Geometry check sheet. Reference: the model listing, model coordinates, mm. A direction names the side the tool comes from. Give positions to 0.01 mm unless a question says otherwise; leave off trailing zeros. Loops run counter-clockwise (first coordinate to the right, second up) from the corner with the lowest first, then second, coordinate; pieces in that order, holes last. Notation, with made-up numbers: (-37, 34.5) -> (-8, 34.5) arc R26 ccw to (-8, 61.5) -> close; hole circle Ø9 at (40, 34). An arc over 180 degrees is marked (long way). Write item = value, one per line.
```python
from build123d import *

# Parameters (mm, degrees)
SKETCH1_W           = 19.05
SKETCH1_H           = 25.4
BOSS_EXTRUDE1_DEPTH = 6.35
SKETCH2_W           = 6.35
SKETCH2_H           = 6.35
CUT_EXTRUDE1_DEPTH  = 7.35
SKETCH6_R           = 0.635
CUT_EXTRUDE2_DEPTH  = 7.35
SKETCH7_R           = 0.635
CUT_EXTRUDE3_DEPTH  = 7.35


with BuildPart() as part:
    # Sketch1 → Boss-Extrude1 (new body)
    with BuildSketch(Plane.XY):
        with Locations((9.525, 12.7)):
            Rectangle(SKETCH1_W, SKETCH1_H)
    extrude(amount=BOSS_EXTRUDE1_DEPTH)

    # Sketch2 → Cut-Extrude1 (cut, through all)
    with BuildSketch(Plane.XY.offset(6.35)):
        with Locations((9.525, 22.225)):
            Rectangle(SKETCH2_W, SKETCH2_H)
    cut_extrude1 = extrude(amount=-CUT_EXTRUDE1_DEPTH, mode=Mode.SUBTRACT)

    # Mirror1: Cut-Extrude1 across plane
    add(cut_extrude1.mirror(Plane.ZX.offset(12.7)), mode=Mode.SUBTRACT)

    # Sketch6 → Cut-Extrude2 (cut, through all)
    with BuildSketch(Plane.XY.offset(6.35)):
        with Locations((3.175, 22.225)):
            Circle(SKETCH6_R)
        with Locations((15.875, 22.225)):
            Circle(SKETCH6_R)
    extrude(amount=-CUT_EXTRUDE2_DEPTH, mode=Mode.SUBTRACT)

    # Sketch7 → Cut-Extrude3 (cut, through all)
    with BuildSketch(Plane(origin=(0, 0, 0), x_dir=(-1, 0, 0), z_dir=(0, 0, -1))):
        with Locations((-15.875, 3.175)):
            Circle(SKETCH7_R)
        with Locations((-3.175, 3.175)):
            Circle(SKETCH7_R)
    extrude(amount=-CUT_EXTRUDE3_DEPTH, mode=Mode.SUBTRACT)


solid = part.part
```
Item 1: Section check B-B, the plane x = 3. Record the cut outline in (y, z), plus the area to 3 significant figures.
Answer:
outline = (0, 0) -> (2.56, 0) -> (2.56, 6.35) -> (0, 6.35) -> close; (3.79, 0) -> (21.61, 0) -> (21.61, 6.35) -> (3.79, 6.35) -> close; (22.84, 0) -> (25.4, 0) -> (25.4, 6.35) -> (22.84, 6.35) -> close
area = 146 mm^2
Item 2: Section check C-C, the plane y = 22.5. Record the cut outline in (x, z).
Answer:
outline = (0, 0) -> (2.6, 0) -> (2.6, 6.35) -> (0, 6.35) -> close; (3.75, 0) -> (6.35, 0) -> (6.35, 6.35) -> (3.75, 6.35) -> close; (12.7, 0) -> (15.3, 0) -> (15.3, 6.35) -> (12.7, 6.35) -> close; (16.45, 0) -> (19.05, 0) -> (19.05, 6.35) -> (16.45, 6.35) -> close
Item 3: Tool access check on faces 4 (the flat face through (9, 19.05, 3)), 5 (the flat face through (6.35, 3, 3)), 6 (the cylindrical face through (16.46, 21.98, 3.22)). Record the directions out of +Z, -Z, +X, -X, +Y, -Y that give a thin tool (end or side, any length) a straight path to the whole face; none if there is none.
Answer:
face_4 = +Z, -Z, +Y
face_5 = +Z, -Z, -Y
face_6 = +Z, -Z
Item 4: Gauge pin test, flat ends, axial feed: pin 1 (2 mm diameter, centred on x = 10.5, z = 2, fed in from +Y); pin 2 (1 mm diameter, centred on x = 3.175, y = 22.225, fed in from +Z). Record the tip position at first contact, or that the pin passes through.
Answer:
pin_1 = 19.05
pin_2 = through
Item 5: Draft check along Y on faces 1 (the cylindrical face through (3.643, 3.604, 3.131)), 2 (the flat face through (12.7, 3, 3)), 3 (the flat face through (9, 6.35, 3)). Enter one of: +Y half, -Y half, draft (parallel to the pull), parting line (faces both ways), or undercut.
Answer:
face_1 = undercut
face_2 = draft
face_3 = -Y half
Item 6: Thickness scan on L1, parallel to X at y = 3.25, z = 0.75; L2, parallel to X at y = 21.5, z = 3.5; L3, parallel to X at y = 22.5, z = 5.5. Record the ranges inside material, lowest first. Write a range as [from, to].
Answer:
L1 = [0, 2.54], [3.81, 6.35], [12.7, 15.24], [16.51, 19.05]
L2 = [0, 6.35], [12.7, 19.05]
L3 = [0, 2.6], [3.75, 6.35], [12.7, 15.3], [16.45, 19.05]
Item 7: Section check D-D, the plane z = 2.25. Record the cut outline in (x, y) (3 decimals), plus the area to 3 significant figures.
Answer:
outline = (0, 0) -> (6.35, 0) -> (6.35, 6.35) -> (12.7, 6.35) -> (12.7, 0) -> (19.05, 0) -> (19.05, 25.4) -> (12.7, 25.4) -> (12.7, 19.05) -> (6.35, 19.05) -> (6.35, 25.4) -> (0, 25.4) -> close; hole circle Ø1.27 at (3.175, 3.175); hole circle Ø1.27 at (3.175, 22.225); hole circle Ø1.27 at (15.875, 3.175); hole circle Ø1.27 at (15.875, 22.225)
area = 398 mm^2
Item 8: Section check A-A, the plane y = 5.5. Record the cut outline in (x, z).
Answer:
outline = (0, 0) -> (6.35, 0) -> (6.35, 6.35) -> (0, 6.35) -> close; (12.7, 0) -> (19.05, 0) -> (19.05, 6.35) -> (12.7, 6.35) -> close
